Input: part model. Units: mm. Frame: model coordinates. Face numbers are marked on the shaded views. Round coordinates to 2 decimals unless told otherwise and drop trailing zeros. Write each loop counter-clockwise with the first axis right and the second up, starting at its lowest first coordinate (ties: lowest second). Pieces come first, ordered by that corner, then holes. Notation, with made-up numbers: (9, 54) -> (57, 54) arc R8 ccw to (57, 66) -> close; hole circle Ø3 at (13, -35). An arc over 180 degrees is marked (long way). Write item = value, one per line.
Autodesk Inventor part; units mm, degrees
ref_plane "YZ Plane" through (0, 0, 0) normal (1, 0, 0) x (0, 1, 0)
ref_plane "XZ Plane" through (0, 0, 0) normal (0, 1, 0) x (-1, 0, 0)
ref_plane "XY Plane" through (0, 0, 0) normal (0, 0, 1) x (1, 0, 0)
sketch "Sketch1" plane through (0, 0, 0) normal (0, 0, 1) x (1, 0, 0)
  line L0 (-15.875, -15.875) -> (15.875, -15.875)
  line L1 (15.875, -15.875) -> (15.875, 15.875)
  line L2 (15.875, 15.875) -> (-15.875, 15.875)
  line L3 (-15.875, 15.875) -> (-15.875, -15.875)
  line L4 (0, 0) -> (0, 6.6196)
  line L5 (-8.6733, 0) -> (9.2317, 0)
  circle A0 centre (-10.16, 10.16) radius 1.8288
  circle A1 centre (10.16, 10.16) radius 1.8288
  circle A2 centre (10.16, -10.16) radius 1.8288
  circle A3 centre (-10.16, -10.16) radius 1.8288
  dimension "d3" = 31.75
  dimension "d4" = 31.75
  dimension "d27" = 20.32
  dimension "d28" = 10.16
  dimension "d29" = 3.6576
  dimension "d30" = 3.6576
  dimension "d31" = 3.6576
  dimension "d32" = 3.6576
  dimension "d35" = 20.32
  dimension "d36" = 10.16
  dimension "d37" = 10.16
extrude "Extrusion1" add sketch "Sketch1" along normal blind 3.175 contours L3 L2 L1 L0 | A0 | A1 | A2 | A3
fillet "Fillet1" radius 1.27 1 edges at (15.875, 15.875, 1.5875)
fillet "Fillet2" radius 1.27 1 edges at (-15.875, 15.875, 1.5875)
fillet "Fillet3" radius 1.27 1 edges at (15.875, -15.875, 1.5875)
fillet "Fillet4" radius 1.27 1 edges at (-15.875, -15.875, 1.5875)
extrude "Extrusion2" cut sketch "Sketch1" along normal through all contours A0 | A1 | A2 | A3
properties part number "MotorMountBottom"
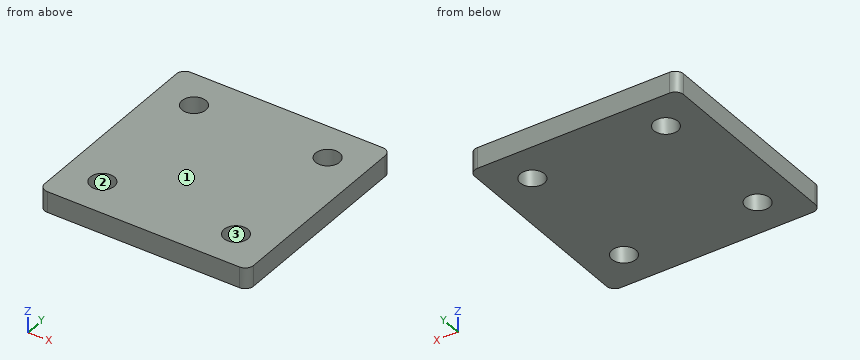
1) Cut plane A-A (y = 10.16). Return the cut outline in (x, z) (3 decimals).
Solutions:
outline = (-15.875, 0) -> (-11.989, 0) -> (-11.989, 3.175) -> (-15.875, 3.175) -> close; (-8.331, 0) -> (8.331, 0) -> (8.331, 3.175) -> (-8.331, 3.175) -> close; (11.989, 0) -> (15.875, 0) -> (15.875, 3.175) -> (11.989, 3.175) -> close
2) Line query: L1, parallel to X at y = -10.16, z = 1.5 (3 decimals); L2, parallel to X at y = 9.5, z = 0.25 (3 decimals). Output: solid intervals per line, ascending. Write a range as from..to.
Solutions:
L1 = -15.875..-11.989, -8.331..8.331, 11.989..15.875
L2 = -15.875..-11.866, -8.454..8.454, 11.866..15.875
3) Draft query along X for the marked faces 1, 2 and 3. Return one class per face: +X half, -X half, draft (parallel to the pull), parting line (faces both ways), or undercut.
Solutions:
face_1 = draft
face_2 = undercut
face_3 = undercut
4) Cut plane C-C (z = 2.5). Return the cut outline in (x, y) (3 decimals).
Solutions:
outline = (-15.875, -14.605) arc R1.27 ccw to (-14.605, -15.875) -> (14.605, -15.875) arc R1.27 ccw to (15.875, -14.605) -> (15.875, 14.605) arc R1.27 ccw to (14.605, 15.875) -> (-14.605, 15.875) arc R1.27 ccw to (-15.875, 14.605) -> close; hole circle Ø3.658 at (-10.16, -10.16); hole circle Ø3.658 at (-10.16, 10.16); hole circle Ø3.658 at (10.16, -10.16); hole circle Ø3.658 at (10.16, 10.16)
